```python
from build123d import *

# Parameters (mm, degrees)
SKETCH1_W                = 200
SKETCH1_H                = 258.87959476
BOSS_EXTRUDE1_DEPTH      = 3
SKETCH2_W                = 200
SKETCH2_H                = 258.87959476
BOSS_EXTRUDE3_DEPTH      = 90
BOSS_EXTRUDE3_DEPTH_BACK = 3
SKETCH3_R                = 2.5
CUT_EXTRUDE2_DEPTH       = 3
SKETCH4_R                = 17.332315934
CUT_EXTRUDE4_DEPTH       = 263.87959476
SKETCH5_R                = 7.5
BOSS_EXTRUDE5_DEPTH      = 10
CUT_EXTRUDE5_REACH       = 239
SKETCH6_R                = 10


with BuildPart() as part:
    # Sketch1 → Boss-Extrude1 (new body)
    with BuildSketch(Plane(origin=(0, 0, 0), x_dir=(-1, 0, 0), z_dir=(0, 0, 1))):
        with Locations((-1.649083583, 6.704740248)):
            Rectangle(SKETCH1_W, SKETCH1_H)
    extrude(amount=BOSS_EXTRUDE1_DEPTH)

    # Sketch2 → Boss-Extrude3 (add, two sides)
    with BuildSketch(Plane.XY.offset(3)) as boss_extrude3_sk:
        Polygon((-100.350916417, 122.735057132), (-100.350916417, -138.144537628), (103.649083583, -138.144537628), (103.649083583, 124.735057132), (-100.350916417, 124.735057132), align=None)
        with Locations((1.649083583, -6.704740248)):
            Rectangle(SKETCH2_W, SKETCH2_H, mode=Mode.SUBTRACT)
    extrude(amount=BOSS_EXTRUDE3_DEPTH)
    extrude(boss_extrude3_sk.sketch, amount=-BOSS_EXTRUDE3_DEPTH_BACK)

    # Sketch3 → Cut-Extrude2 (cut)
    with BuildSketch(Plane(origin=(0, 0, 0), x_dir=(-1, 0, 0), z_dir=(0, 0, -1))):
        with Locations((41.514444489, -9.336870594)):
            Circle(SKETCH3_R)
        with Locations((-9.485555511, 35.263129406)):
            Circle(SKETCH3_R)
        with Locations((-9.485555511, -53.936870594)):
            Circle(SKETCH3_R)
        with Locations((-46.985555511, -20.636870594)):
            Circle(SKETCH3_R)
    extrude(amount=-CUT_EXTRUDE2_DEPTH, mode=Mode.SUBTRACT)

    # Sketch4 → Cut-Extrude4 (cut, through all)
    with BuildSketch(Plane.XZ.offset(138.144537628)):
        with Locations((1.649062898, 92.934091246)):
            Circle(SKETCH4_R)
    extrude(amount=-CUT_EXTRUDE4_DEPTH, mode=Mode.SUBTRACT)

    # Sketch5 → Boss-Extrude5 (add)
    with BuildSketch(Plane.XY.offset(93)):
        with BuildLine():
            Line((103.649083583, 8.295259752), (103.649083583, -6.704740248))
            Line((103.649083583, -6.704740248), (103.649083583, -21.704740248))
            Line((103.649083583, -21.704740248), (121.649083583, -21.704740248))
            ThreePointArc((121.649083583, -21.704740248), (136.649083583, -6.704740248), (121.649083583, 8.295259752))
            Line((121.649083583, 8.295259752), (103.649083583, 8.295259752))
        make_face()
        with Locations((121.649083583, -6.704740248)):
            Circle(SKETCH5_R, mode=Mode.SUBTRACT)
        with BuildLine():
            Line((-100.350916417, -21.704740248), (-100.350916417, -6.704740248))
            Line((-100.350916417, -6.704740248), (-100.350916417, 8.295259752))
            Line((-100.350916417, 8.295259752), (-118.350916417, 8.295259752))
            ThreePointArc((-118.350916417, 8.295259752), (-133.350916417, -6.704740248), (-118.350916417, -21.704740248))
            Line((-118.350916417, -21.704740248), (-100.350916417, -21.704740248))
        make_face()
        with Locations((-118.350916417, -6.704740248)):
            Circle(SKETCH5_R, mode=Mode.SUBTRACT)
    extrude(amount=-BOSS_EXTRUDE5_DEPTH)

    # Sketch6 → Cut-Extrude5 (cut, up to next)
    with BuildSketch(Plane.ZY.offset(100.350916417), mode=Mode.PRIVATE) as cut_extrude5_sk1:
        with Locations((18.364873633, 57.542228563)):
            Circle(SKETCH6_R)
    cut_extrude5_tool1 = extrude(cut_extrude5_sk1.sketch, amount=-CUT_EXTRUDE5_REACH, mode=Mode.PRIVATE) & part.part
    add(cut_extrude5_tool1.solids().sort_by_distance((-100.350916, 57.542229, 18.364874))[0], mode=Mode.SUBTRACT)


solid = part.part
```
Work out the finished part from the listing and answer in its coordinate system (mm). A direction names the side the tool comes from. Give positions to 0.01 mm unless a question says otherwise; leave off trailing zeros. Loops run counter-clockwise (first coordinate to the right, second up) from the corner with the lowest first, then second, coordinate; pieces in that order, holes last. Notation, with made-up numbers: M -13.5,89.5 L 43.5,89.5 A20 cw 43.5,118.5 Z; hole C -26,-36.75 d9. An arc over 180 degrees is marked long. One line per item, written item: value. Start each with the question number.
1. Find section C-C (y = 86). Give the vertices of the cut face in (x, z).
2. Find section A-A (z = 45). Give the vertices of the cut face in (x, y), and give its area (3 significant figures).
3. Find the intervals of material crossed by probe 1 along Y at (x, z) = (-87, 48); probe 2 along X at (y, z) = (71.5, 5); probe 3 along Z at (x, y) = (19, -53.5), in increasing order.
4. Each of these flat-tipped pins is pushed along its axis until it touches: P1, Ø6, axis at x = 64.5, y = 55.5, coming from the +Z side; P2, Ø5, axis at x = 109.5, z = 88.5, coming from the -Y side; P3, Ø11, axis at x = -106.5, z = 85.5, coming from the +Y side. Where does it stop, or does it pass through?
5. Which of the six approach directions +Z, -Z, +X, -X, +Y, -Y give full straight-line access (tool end or side, diameter ignored) to faces 1 (the face through (112, -6, 93)), 2 (the face through (-109, 8.295, 88)), 3 (the face through (0, -5, 0)), 4 (the face through (0, 122.735, 47)), 5 (the face through (-109, -21.705, 88))?
6. Find section B-B (x = 94.5). Give the vertices of the cut face in (y, z), and give its area (3 significant figures).
7. Find section D-D (z = 79.5). Give the vertices of the cut face in (x, y), and give its area (3 significant figures).
8. Determine the mould class of faces 6 (the face through (113, 8.295, 88)), 7 (the face through (-110, -6, 93)), 8 (the face through (-99.36, 48.67, 22.98)) for opening direction Z: released by +Z, released by -Z, zero draft, split by the parting line, or undercut.
Reported:
1. outline: M -100.35,0 L 103.65,0 L 103.65,93 L 101.65,93 L 101.65,3 L -98.35,3 L -98.35,93 L -100.35,93 Z
2. outline: M -100.35,-138.14 L 103.65,-138.14 L 103.65,124.74 L -100.35,124.74 Z; hole M -98.35,-136.14 L 101.65,-136.14 L 101.65,122.74 L -98.35,122.74 Z
2. area: 1,850 mm²
3. probe 1: y = -138.14 to -136.14, 122.74 to 124.74
3. probe 2: x = -100.35 to -98.35, 101.65 to 103.65
3. probe 3: z = 0 to 3
4. P1: stops at z = 3
4. P2: stops at y = -21.7
4. P3: stops at y = 8.3
5. face 1: +Z, +X, -X, +Y, -Y
5. face 2: +Z, -Z, -X, +Y
5. face 3: -Z, +X, -X, +Y, -Y
5. face 4: +Z
5. face 5: +Z, -Z, -X, -Y
6. outline: M -138.14,0 L 124.74,0 L 124.74,93 L 122.74,93 L 122.74,3 L -136.14,3 L -136.14,93 L -138.14,93 Z
6. area: 1,150 mm²
7. outline: M -100.35,-138.14 L -9.3,-138.14 L -9.3,-136.14 L -98.35,-136.14 L -98.35,122.74 L -9.3,122.74 L -9.3,124.74 L -100.35,124.74 Z; M 12.6,-138.14 L 103.65,-138.14 L 103.65,124.74 L 12.6,124.74 L 12.6,122.74 L 101.65,122.74 L 101.65,-136.14 L 12.6,-136.14 Z
7. area: 1,760 mm²
8. face 6: zero draft
8. face 7: released by +Z
8. face 8: undercut
